Geometry check sheet. Reference: the model listing, model coordinates, mm. A direction names the side the tool comes from. Give positions to 0.01 mm unless a question says otherwise; leave off trailing zeros. Write each loop counter-clockwise with the first axis right and the second up, starting at its lowest first coordinate (ties: lowest second). Pieces come first, ordered by that corner, then holes.
(1) Tool access check on faces 4 (the flat face through (57, 15, -58.42)), 5 (the cylindrical face through (6.524, 28.074, -6.741)), 6 (the flat face through (58, 17.78, -31)), 7 (the flat face through (18, 51.943, -35)). Record the directions out of +Z, -Z, +X, -X, +Y, -Y that give a thin tool (end or side, any length) a straight path to the whole face; none if there is none.
(2) Depth check by flat-ended pin: P1, Ø4.5, axis at x = 59, z = -39.5, coming from the -Y side; P2, Ø10.5, axis at x = 15.5, z = -25.5, coming from the +Y side; P3, Ø13.5, axis at x = 97.282, z = -30.48, coming from the +Y side. Enter the tip coordinate at first touch or a pass-through.
(3) Cross-section at A-A (y = 36). Record the boundary of the cut face in (x, z) (3 decimals).
(4) Cross-section at C-C (y = 7.5). Record the boundary of the cut face in (x, z), and give its area (3 significant figures).
(5) Mould release check, pull along X, two halves, no side actions. Record for faces 1 (the flat face through (107.83, 9.63, -53.35)), 2 (the flat face through (21, 0, -34)), 3 (the flat face through (105.63, 9.18, -51.17)): +X half, -X half, draft (parallel to the pull), parting line (faces both ways), or undercut.
(6) Cross-section at B-B (z = -30.48). Count the separate pieces of the cut face and the enclosed holes in it, and give its area (3 significant figures).
(7) Thickness scan on line 1 along X through (y, z) = (29, -54) (3 decimals); line 2 along Z through (x, y) = (92, 35); line 3 along Z through (x, y) = (93.5, 3.5). Record the ranges inside material, lowest first.
(8) Cross-section at D-D (x = 17.78). Record the boundary of the cut face in (y, z) (3 decimals), and give its area (3 significant figures).
```python
from build123d import *

# Parameters (mm, degrees)
SKETCH1_W                                = 115.062
SKETCH1_H                                = 60.96
BOSS_EXTRUDE1_DEPTH                      = 57.912
SKETCH3_W                                = 32.512
SKETCH3_H                                = 40.132
CUT_EXTRUDE1_DEPTH                       = 79.502
FILLET1_R                                = 16.51
FILLET2_R                                = 8.89
CBORE_FOR_5_16_HEX_HEAD_BOLT1_AT_2_COUNT = 2
CBORE_FOR_5_16_HEX_HEAD_BOLT1_AT_2_PITCH = 79.502
MIRROR1_START                            = -43.619425251
MIRROR1_OUTLINE_W                        = 33
MIRROR1_OUTLINE_H                        = 39
MIRROR1_DEPTH                            = 13.631070391
SHELL1_T                                 = -2.54


# Read off the part's stored shape, not the designer's step: Mirror1
with BuildPart() as part:
    # Sketch1 → Boss-Extrude1 (new body)
    with BuildSketch(Plane(origin=(0, 0, 0), x_dir=(1, 0, 0), z_dir=(0, 1, 0))):
        with Locations((57.531, 30.48)):
            Rectangle(SKETCH1_W, SKETCH1_H)
    extrude(amount=BOSS_EXTRUDE1_DEPTH)

    # Sketch3 → Cut-Extrude1 (cut)
    with BuildSketch(Plane(origin=(0, 0, -60.96), x_dir=(-1, 0, 0), z_dir=(0, 0, -1))):
        with Locations((-57.531, 37.846)):
            Rectangle(SKETCH3_W, SKETCH3_H)
    extrude(amount=-CUT_EXTRUDE1_DEPTH, mode=Mode.SUBTRACT)

    # Fillet1
    fillet1_edges = [part.edges().sort_by_distance(p)[0] for p in [
        (115.062, 28.956, 0),
        (0, 28.956, 0),
    ]]
    fillet(fillet1_edges, radius=FILLET1_R)

    # Fillet2
    fillet2_edges = [part.edges().sort_by_distance(p)[0] for p in [
        (73.787, 57.912, -30.48),
        (41.275, 57.912, -30.48),
        (41.275, 17.78, -30.48),
        (73.787, 17.78, -30.48),
    ]]
    fillet(fillet2_edges, radius=FILLET2_R)

    # Sketch5 → CBORE for 5/16 Hex Head Bolt1 (revolve, cut)
    with BuildSketch(Plane(origin=(17.78, 57.912, -30.48), x_dir=(0, 0, 1), z_dir=(1, 0, 0))):
        Polygon((0, 0), (0, 57.912), (4.2164, 57.912), (4.2164, 5.969), (10.31875, 5.969), (10.31875, 0.532828266), (10.95375, 0), align=None)
    cbore_for_5_16_hex_head_bolt1 = revolve(axis=Axis((17.78, 64.262, -30.48), (0, -1, 0)), mode=Mode.SUBTRACT)

    # CBORE for 5/16 Hex Head Bolt1 at 2: CBORE for 5/16 Hex Head Bolt1 ×2
    with Locations(*[(i * CBORE_FOR_5_16_HEX_HEAD_BOLT1_AT_2_PITCH, 0, 0) for i in range(1, CBORE_FOR_5_16_HEX_HEAD_BOLT1_AT_2_COUNT)]):
        add(cbore_for_5_16_hex_head_bolt1, mode=Mode.SUBTRACT)

    # SurfaceCut1
    split(bisect_by=Plane(origin=(49.231296, -41.02608, -65.641728), x_dir=(0.8438009243891594, 0.2844272778839867, 0.45508364461437806), z_dir=(-0.5366563145999497, 0.44721359549995837, 0.7155417527999325)), keep=Keep.TOP)

    # Mirror1 outline → Mirror1 (cut)
    with BuildSketch(Plane(origin=(0, 0, 0), x_dir=(0.8438009243891591, -0.284427277883987, -0.4550836446143786), z_dir=(0.5366563145999501, 0.4472135954999582, 0.7155417527999323)).offset(MIRROR1_START)):
        with Locations((34.5, 40.5)):
            Rectangle(MIRROR1_OUTLINE_W, MIRROR1_OUTLINE_H)
    extrude(amount=MIRROR1_DEPTH, mode=Mode.SUBTRACT)

    # Shell1
    shell1_openings = [part.faces().sort_by_distance(p)[0] for p in [
        (57.531, 0, -29.124585382),
    ]]
    offset(amount=SHELL1_T, openings=shell1_openings, kind=Kind.INTERSECTION)


solid = part.part
```
Reply:
1. face 4: none
1. face 5: -Y
1. face 6: +Z, -Z, +Y
1. face 7: +Y
2. P1: stops at y = 15.24
2. P2: stops at y = 57.72
2. P3: stops at y = 51.94
3. outline: (0, -60.96) - (41.275, -60.96) - (41.275, 0) - (16.51, 0) arc R16.51 ccw to (0, -16.51) - close; circle Ø13.513 at (17.78, -30.48); (73.787, -60.96) - (115.062, -60.96) - (115.062, -16.51) arc R16.51 ccw to (98.552, 0) - (73.787, 0) - close; circle Ø13.513 at (97.282, -30.48); hole (2.54, -58.42) - (38.735, -58.42) - (38.735, -2.54) - (16.51, -2.54) arc R13.97 ccw to (2.54, -16.51) - close; hole circle Ø8.433 at (17.78, -30.48); hole (76.327, -58.42) - (112.522, -58.42) - (112.522, -16.51) arc R13.97 ccw to (98.552, -2.54) - (76.327, -2.54) - close; hole circle Ø8.433 at (97.282, -30.48)
4. outline: (0, -46.6) - (19.15, -60.96) - (95.91, -60.96) - (115.06, -46.6) - (115.06, -16.51) arc R16.51 ccw to (98.55, 0) - (16.51, 0) arc R16.51 ccw to (0, -16.51) - close; circle Ø13.51 at (17.78, -30.48); circle Ø13.51 at (97.28, -30.48); hole (2.54, -44.95) - (20.5, -58.42) - (94.57, -58.42) - (112.52, -44.95) - (112.52, -16.51) arc R13.97 ccw to (98.55, -2.54) - (16.51, -2.54) arc R13.97 ccw to (2.54, -16.51) - close; hole circle Ø8.43 at (17.78, -30.48); hole circle Ø8.43 at (97.28, -30.48)
4. area: 977 mm2
5. face 1: +X half
5. face 2: draft
5. face 3: undercut
6. separate pieces: 3
6. enclosed holes: 0
6. area: 1,260 mm2
7. line 1: x = 0 to 2.54, 38.735 to 41.275, 73.787 to 76.327, 112.522 to 115.062
7. line 2: z = -60.96 to -58.42, -34.69 to -26.27, -2.54 to 0
7. line 3: z = -60.27 to -56.72, -36.08 to -32.34, -28.62 to -24.88, -2.54 to 0
8. outline: (0, -55.245) - (9.144, -60.96) - (57.912, -60.96) - (57.912, -41.434) - (57.379, -40.799) - (51.943, -40.799) - (51.943, -34.696) - (0, -34.696) - (0, -37.236) - (49.403, -37.236) - (49.403, -43.339) - (55.372, -43.339) - (55.372, -58.42) - (10.76, -58.42) - (0, -51.695) - close; (0, -26.264) - (51.943, -26.264) - (51.943, -20.161) - (57.379, -20.161) - (57.912, -19.526) - (57.912, 0) - (0, 0) - (0, -2.54) - (55.372, -2.54) - (55.372, -17.621) - (49.403, -17.621) - (49.403, -23.724) - (0, -23.724) - close
8. area: 706 mm2
